from build123d import *

# Parameters (mm, degrees)
BOX_W           = 20
BOX_H           = 5
BOX_DEPTH       = 5
CYLINDER_R      = 10
CYLINDER_DEPTH  = 8
POCKET_DEPTH    = 6
SKETCH001_R     = 10
PAD_DEPTH       = 2
SKETCH002_R     = 3.4
POCKET001_DEPTH = 2
POCKET002_DEPTH = 20.001
SKETCH004_R     = 15
SKETCH004_R_2   = 10
POCKET003_DEPTH = 15.001


with BuildPart() as attachpart:
    # Box → Box (new body)
    with BuildSketch(Plane(origin=(-10, -2.5, 10), x_dir=(1, 0, 0), z_dir=(0, 0, 1))):
        with Locations((10, 2.5)):
            Rectangle(BOX_W, BOX_H)
    extrude(amount=BOX_DEPTH)


with BuildPart() as attachbody:
    # Cylinder → Cylinder (new body)
    with BuildSketch(Plane.XY):
        Circle(CYLINDER_R)
    extrude(amount=CYLINDER_DEPTH)

    # Sketch (on Face2 of BaseFeature) → Pocket (cut)
    with BuildSketch(Plane.XY.offset(8)):
        Polygon((3.45, -5.975575), (6.9, 0), (3.45, 5.975575), (-3.45, 5.975575), (-6.9, 0), (-3.45, -5.975575), align=None)
    extrude(amount=-POCKET_DEPTH, mode=Mode.SUBTRACT)

    # Sketch001 (on Face2 of Pocket) → Pad (join)
    with BuildSketch(Plane.XY.offset(8)):
        Circle(SKETCH001_R)
    extrude(amount=PAD_DEPTH)

    # Sketch002 (on Face3 of Pad) → Pocket001 (cut)
    with BuildSketch(Plane(origin=(0, 0, 0), x_dir=(1, 0, 0), z_dir=(0, 0, -1))):
        Circle(SKETCH002_R)
    extrude(amount=-POCKET001_DEPTH, mode=Mode.SUBTRACT)

    # Fusion: union AttachPart
    add(attachpart.part)

    # Sketch003 (on Face11 of BaseFeature001) → Pocket002 (cut, through all)
    with BuildSketch(Plane.YZ.offset(10)):
        Polygon((2.3, 15), (2.5, 15), (2.5, 10), (1.05, 10), align=None)
        Polygon((-2.5, 15), (-2.3, 15), (-1.05, 10), (-2.5, 10), align=None)
    extrude(amount=-POCKET002_DEPTH, mode=Mode.SUBTRACT)

    # Sketch004 (on Face3 of Pocket002) → Pocket003 (cut, through all)
    with BuildSketch(Plane(origin=(0, 0, 0), x_dir=(1, 0, 0), z_dir=(0, 0, -1))):
        Circle(SKETCH004_R)
        Circle(SKETCH004_R_2, mode=Mode.SUBTRACT)
    extrude(amount=-POCKET003_DEPTH, mode=Mode.SUBTRACT)


solid = attachbody.part
Model file for the job. Use its own axes, mm. A direction names the side the tool comes from. Round coordinates to 2 decimals unless told otherwise and drop trailing zeros. Loops run counter-clockwise (first coordinate to the right, second up) from the corner with the lowest first, then second, coordinate; pieces in that order, holes last. Notation, with made-up numbers: (69, 23.25) -> (114, 23.25) arc R17 cw to (114, 46.25) -> close; hole circle Ø2 at (72.5, 10). An arc over 180 degrees is marked (long way). Answer as CSV lines item,"result". Start each with the question number.
1) Slice it at A-A (z = 3.5). List the corners of the cut face in (x, y).
2) Slice it at D-D (z = 9.5). List the corners of the cut face in (x, y), plus the area to 3 significant figures.
3) Mould opens along X. For faces 1 (the face through (-5.15, 3.03, 5.04)), 2 (the face through (0, 5, 10)), 3 (the face through (-10, 0, 6)) say: +X half, -X half, draft (parallel to the pull), parting line (faces both ways), or undercut.
4) Slice it at C-C (x = 0). List the corners of the cut face in (y, z), plus the area to 3 significant figures.
5) Slice it at B-B (x = 4.75). List the corners of the cut face in (y, z), plus the area to 3 significant figures.
6) Tool access for faces 4 (the face through (0.139, -1.684, 12.535)), 5 (the face through (0, -5.976, 5)), 6 (the face through (0.139, 1.666, 12.465)), 7 (the face through (0, 0, 15)), 8 (the face through (-0.74, 3.32, 0.99)): list every direction of +Z, -Z, +X, -X, +Y, -Y with a clear straight run to the whole face (end or side of a thin tool).
7) Pin check, flat tips, straight feed: P1, Ø3, axis at x = 2.5, z = 10.5, coming from the -Y side; P2, Ø8, axis at y = -7.5, z = 2, coming from the +X side; P3, Ø1, axis at y = 8, z = 7, coming from the -X side. Stop position of each tip, or through.
8) Probe line 1 along Y through (x, z) = (0, 0.55); line 2 along Y through (x, z) = (0.25, 3.5). List the from-to ranges inside material, lowest first.
Filled in:
1,outline,"circle Ø20 at (0, 0); hole (-6.9, 0) -> (-3.45, -5.98) -> (3.45, -5.98) -> (6.9, 0) -> (3.45, 5.98) -> (-3.45, 5.98) -> close"
2,outline,"circle Ø20 at (0, 0)"
2,area,"314 mm2"
3,face 1,"undercut"
3,face 2,"draft"
3,face 3,"parting line"
4,outline,"(-10, 0) -> (-3.4, 0) -> (-3.4, 2) -> (-5.98, 2) -> (-5.98, 8) -> (5.98, 8) -> (5.98, 2) -> (3.4, 2) -> (3.4, 0) -> (10, 0) -> (10, 10) -> (1.05, 10) -> (2.3, 15) -> (-2.3, 15) -> (-1.05, 10) -> (-10, 10) -> close"
4,area,"131 mm2"
5,outline,"(-8.8, 0) -> (8.8, 0) -> (8.8, 10) -> (1.05, 10) -> (2.3, 15) -> (-2.3, 15) -> (-1.05, 10) -> (-8.8, 10) -> close; hole (-3.72, 2) -> (3.72, 2) -> (3.72, 8) -> (-3.72, 8) -> close"
5,area,"148 mm2"
6,face 4,"+X, -X, -Y"
6,face 5,"none"
6,face 6,"+X, -X, +Y"
6,face 7,"+Z, +X, -X, +Y, -Y"
6,face 8,"-Z"
7,P1,"stops at y = -9.94"
7,P2,"stops at x = 9.37"
7,P3,"stops at x = -6.61"
8,line 1,"y = -10 to -3.4, 3.4 to 10"
8,line 2,"y = -10 to -5.98, 5.98 to 10"
